from build123d import *

# Parameters (mm, degrees)
SKETCH1_R           = 30.851139148
BOSS_EXTRUDE1_DEPTH = 2
DOME1_FACE_RADIUS   = 30.851139148
DOME1_HEIGHT        = 10
DOME2_FACE_RADIUS   = 30.851139148
DOME2_HEIGHT        = 10


with BuildPart() as part:
    # Sketch1 → Boss-Extrude1 (new body)
    with BuildSketch(Plane(origin=(0, 0, 0), x_dir=(0, 0, -1), z_dir=(1, 0, 0))):
        Circle(SKETCH1_R)
    extrude(amount=BOSS_EXTRUDE1_DEPTH)

    # Dome1: a dome of height H over a round flat face of radius A is a cap of a sphere of radius (A * A + H * H) / (2 * H)
    dome1_r = (DOME1_FACE_RADIUS * DOME1_FACE_RADIUS + DOME1_HEIGHT * DOME1_HEIGHT) / (2 * DOME1_HEIGHT)
    dome1_base = Plane((2, 0, 0), z_dir=(1, 0, 0))
    with Locations(dome1_base.offset(DOME1_HEIGHT - dome1_r)):
        dome1_ball = Sphere(dome1_r, mode=Mode.PRIVATE)
    add(split(dome1_ball, bisect_by=dome1_base, keep=Keep.TOP, mode=Mode.PRIVATE))

    # Dome2: a dome of height H over a round flat face of radius A is a cap of a sphere of radius (A * A + H * H) / (2 * H)
    dome2_r = (DOME2_FACE_RADIUS * DOME2_FACE_RADIUS + DOME2_HEIGHT * DOME2_HEIGHT) / (2 * DOME2_HEIGHT)
    dome2_base = Plane((0, 0, 0), z_dir=(-1, 0, 0))
    with Locations(dome2_base.offset(DOME2_HEIGHT - dome2_r)):
        dome2_ball = Sphere(dome2_r, mode=Mode.PRIVATE)
    add(split(dome2_ball, bisect_by=dome2_base, keep=Keep.TOP, mode=Mode.PRIVATE))


solid = part.part
Check sheet for the modelled part. Datum: model origin and axes. Units: mm. Round coordinates to 2 decimals unless told otherwise and drop trailing zeros. Order: outer loops, then holes, each group sorted by start corner. A loop starts at its lowest first (then second) coordinate and runs counter-clockwise, first axis right, second up. Notation, with made-up numbers: M -17.75,62 L 6.25,62 A11 ccw 6.25,73 Z; hole C 28,75 d1. An arc over 180 degrees is marked long. One line per item, written item: value. Start each with the question number.
1. Section check A-A on z = 0. Enter the section's corners in (x, y).
2. Section check D-D on x = -8. Enter the section's corners in (y, z), and give its area (3 significant figures).
3. Gauge pin test, flat ends, axial feed: P1, Ø8, axis at x = 4, z = -11.5, coming from the +Y side; P2, Ø3, axis at y = -1.5, z = -3.5, coming from the -X side; P3, Ø10, axis at x = 2, z = -20, coming from the +Y side. Record the tip position at first contact, or that the pin passes through.
4. Scan lines: line 1 along Y through (x, z) = (0.5, -0.5); line 2 along Y through (x, z) = (-5, 7.5); line 3 along X through (y, z) = (-0.5, -23). Record each from-to range of solid material in increasing order.
5. Section check C-C on x = 9.25. Enter the section's corners in (y, z), and give its area (3 significant figures).
6. Section check B-B on y = -8.5. Enter the section's corners in (x, z), and give its area (3 significant figures).
Results found:
1. outline: M 0,-30.85 L 2,-30.85 A52.59 ccw 2,30.85 L 0,30.85 A52.59 ccw Z
2. outline: C 0,0 d28.73
2. area: 648 mm^2
3. P1: y = 29.79
3. P2: x = -9.95
3. P3: y = 26.96
4. line 1: -30.85 to 30.85
4. line 2: -21.09 to 21.09
4. line 3: -4.7 to 6.7
5. outline: C 0,0 d33.57
5. area: 885 mm^2
6. outline: M 0,-29.66 L 2,-29.66 A51.9 ccw 2,29.66 L 0,29.66 A51.9 ccw Z
6. area: 869 mm^2
